Geometry: see drawing. Coordinates: mm, zero at the bounding-box minimum. Round coordinates to 2 decimals unless told otherwise and drop trailing zeros. Write each loop counter-clockwise with the first axis right and the second up, starting at its lowest first coordinate (ties: lowest second). Pieces come first, ordered by that corner, then holes. Notation, with made-up numbers: (19.25, 89.25) -> (38.25, 89.25) arc R33 cw to (38.25, 117.25) -> close; hole circle Ø7 at (-16.5, 58.5). An arc over 180 degrees is marked (long way). Write item = value, one per line. Start each with the question number.
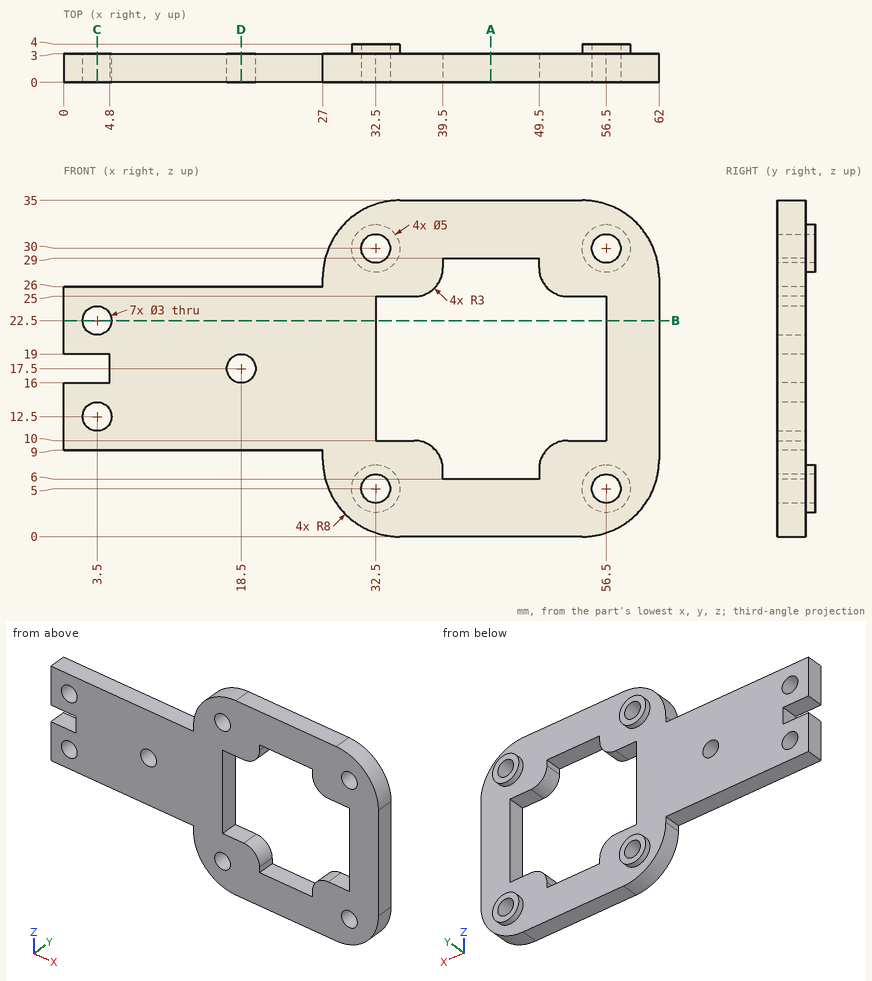
1. Section A-A (x = 44.5). Output: boundary loops of the cut face in (y, z), then the cut area to 3 significant figures.
2. Section B-B (z = 22.5). Output: boundary loops of the cut face in (x, y).
3. Line query: line 1 along X through (y, z) = (1.7, 22.5); line 2 along X through (y, z) = (2.1, 17.5); line 3 along Z through (x, y) = (43, 1.75). Output: solid intervals per line, ascending.
4. Section D-D (x = 18.5). Output: boundary loops of the cut face in (y, z), then the cut area to 3 significant figures.
5. Pin query (flat end, axial travel): P1, Ø8, axis at x = 44, z = 13.5, coming from the -Y side; P2, Ø2, axis at x = 29, y = 1, coming from the -Z side (3 decimals); P3, Ø0.8, axis at y = 1, z = 6.5, coming from the -X side; P4, Ø12, axis at x = 39.5, z = 15, coming from the +Y side. Return the tip coordinate at first contact, or that it passes through.
6. Section C-C (x = 3.5). Output: boundary loops of the cut face in (y, z), then the cut area to 3 significant figures.
Check sheet entries:
q1.outline = (0, 0) -> (3, 0) -> (3, 6) -> (0, 6) -> close; (0, 29) -> (3, 29) -> (3, 35) -> (0, 35) -> close
q1.area = 36.0 mm2
q2.outline = (0, 0) -> (2, 0) -> (2, 3) -> (0, 3) -> close; (5, 0) -> (32.5, 0) -> (32.5, 3) -> (5, 3) -> close; (56.5, 0) -> (62, 0) -> (62, 3) -> (56.5, 3) -> close
q3.line_1 = 0 to 2, 5 to 32.5, 56.5 to 62
q3.line_2 = 4.8 to 17, 20 to 32.5, 56.5 to 62
q3.line_3 = 0 to 6, 29 to 35
q4.outline = (0, 9) -> (3, 9) -> (3, 16) -> (0, 16) -> close; (0, 19) -> (3, 19) -> (3, 26) -> (0, 26) -> close
q4.area = 42.0 mm2
q5.P1 = through
q5.P2 = 1.755
q5.P3 = 27.08
q5.P4 = 3
q6.outline = (0, 9) -> (3, 9) -> (3, 11) -> (0, 11) -> close; (0, 14) -> (3, 14) -> (3, 16) -> (0, 16) -> close; (0, 19) -> (3, 19) -> (3, 21) -> (0, 21) -> close; (0, 24) -> (3, 24) -> (3, 26) -> (0, 26) -> close
q6.area = 24.0 mm2
